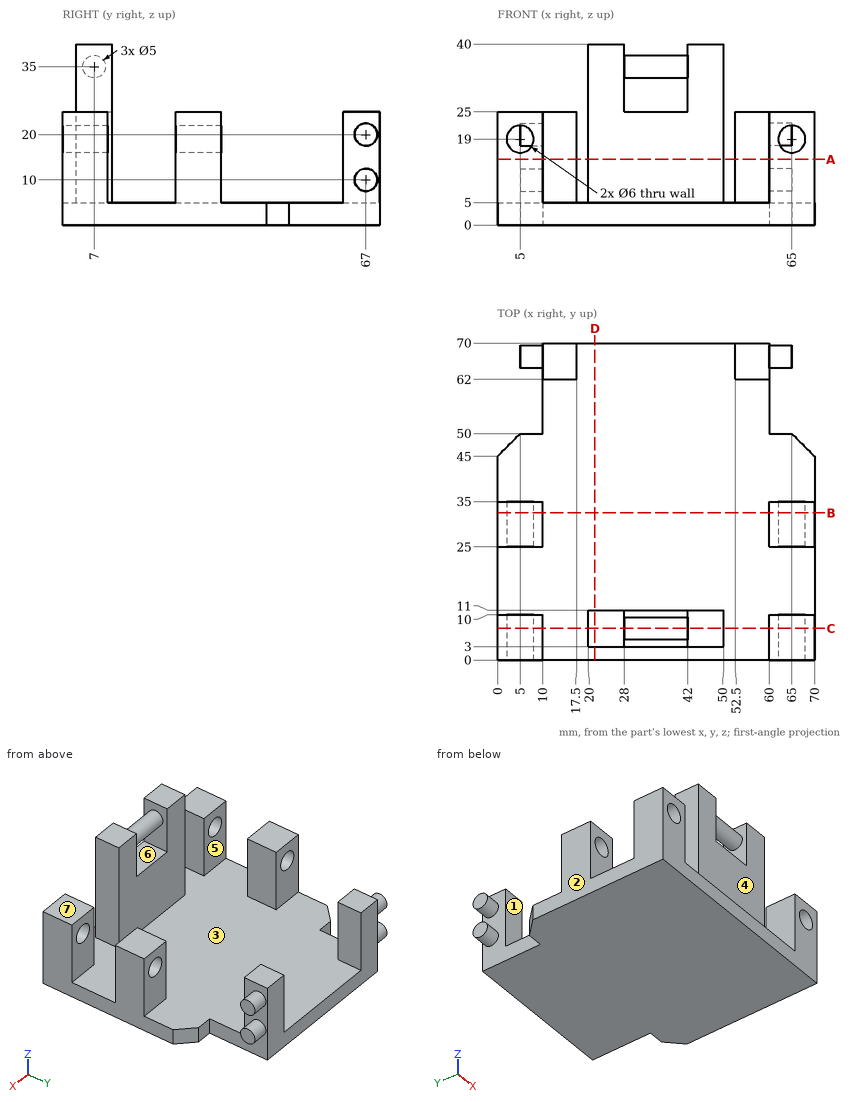
Here's the drawing with two shaded views (mm, measured from the low corner). I have some questions. A direction names the side the tool comes from. Coordinates: 2 decimals unless noted, no trailing zeros. Loops run counter-clockwise (first coordinate to the right, second up) from the corner with the lowest first, then second, coordinate; pieces in that order, holes last.
Item 1: Please list where these lines run through material, in increasing order: L1, parallel to Z at x = 65, y = 2; L2, parallel to X at y = 27, z = 23; L3, parallel to Y at x = 3.5, z = 7.
Answers below:
L1: z = 0 to 16, 22 to 25
L2: x = 0 to 10, 60 to 70
L3: y = 0 to 10, 25 to 35
Item 2: I'm going to push flat-ended pins straight in: pin 1 (6.5 mm diameter, centred on x = 36.5, y = 7.5, fed in from +Z); pin 2 (8 mm diameter, centred on x = 65, z = 13.5, fed in from +Y); pin 3 (8 mm diameter, centred on x = 4, y = 29, fed in from +Z). Where does each tip first touch, or does it pass through?
Answers below:
pin 1: stops at z = 37.5
pin 2: stops at y = 69.5
pin 3: stops at z = 25
Item 3: Suppose I cut it at B-B (y = 32.5). Please give me the cut outline in (x, z), then the cut area to 3 significant figures.
Answers below:
outline: (0, 0) - (70, 0) - (70, 25) - (60, 25) - (60, 5) - (10, 5) - (10, 25) - (0, 25) - close; hole circle Ø6 at (5, 19); hole circle Ø6 at (65, 19)
area: 693 mm2
Item 4: Which directions (+Z, -Z, +X, -X, +Y, -Y) give clear straight access to the entire face, cutting with the end or side of a thin tool? Please do the marked faces 4, 5, 6 and 7.
Answers below:
face 4: +Z, -Y
face 5: +Z, -X
face 6: +Y, -Y
face 7: +Z, +X, +Y, -Y
Item 5: Suppose I cut it at D-D (x = 21.5). Please give me the cut outline in (y, z).
Answers below:
outline: (0, 0) - (70, 0) - (70, 5) - (11, 5) - (11, 40) - (3, 40) - (3, 5) - (0, 5) - close
Item 6: Suppose I cut it at A-A (z = 14.5). Please give me the cut outline in (x, y), then the cut area to 3 significant figures.
Answers below:
outline: (0, 0) - (10, 0) - (10, 10) - (0, 10) - close; (0, 25) - (10, 25) - (10, 35) - (0, 35) - close; (10, 62) - (17.5, 62) - (17.5, 70) - (10, 70) - close; (20, 3) - (50, 3) - (50, 11) - (20, 11) - close; (52.5, 62) - (60, 62) - (60, 70) - (52.5, 70) - close; (60, 0) - (70, 0) - (70, 10) - (60, 10) - close; (60, 25) - (70, 25) - (70, 35) - (60, 35) - close
area: 760 mm2
Item 7: Suppose I cut it at C-C (y = 7). Please give me the cut outline in (x, z).
Answers below:
outline: (0, 0) - (70, 0) - (70, 25) - (60, 25) - (60, 5) - (50, 5) - (50, 40) - (42, 40) - (42, 37.5) - (28, 37.5) - (28, 40) - (20, 40) - (20, 5) - (10, 5) - (10, 25) - (0, 25) - close; hole circle Ø6 at (5, 19); hole (28, 25) - (42, 25) - (42, 32.5) - (28, 32.5) - close; hole circle Ø6 at (65, 19)
Item 8: If we mould it in two halves opening along X, with no side actions, what happens to the marked faces 1, 2 and 3? For each: released by +X, released by -X, zero draft, split by the parting line, or undercut.
Answers below:
face 1: zero draft
face 2: released by -X
face 3: undercut
